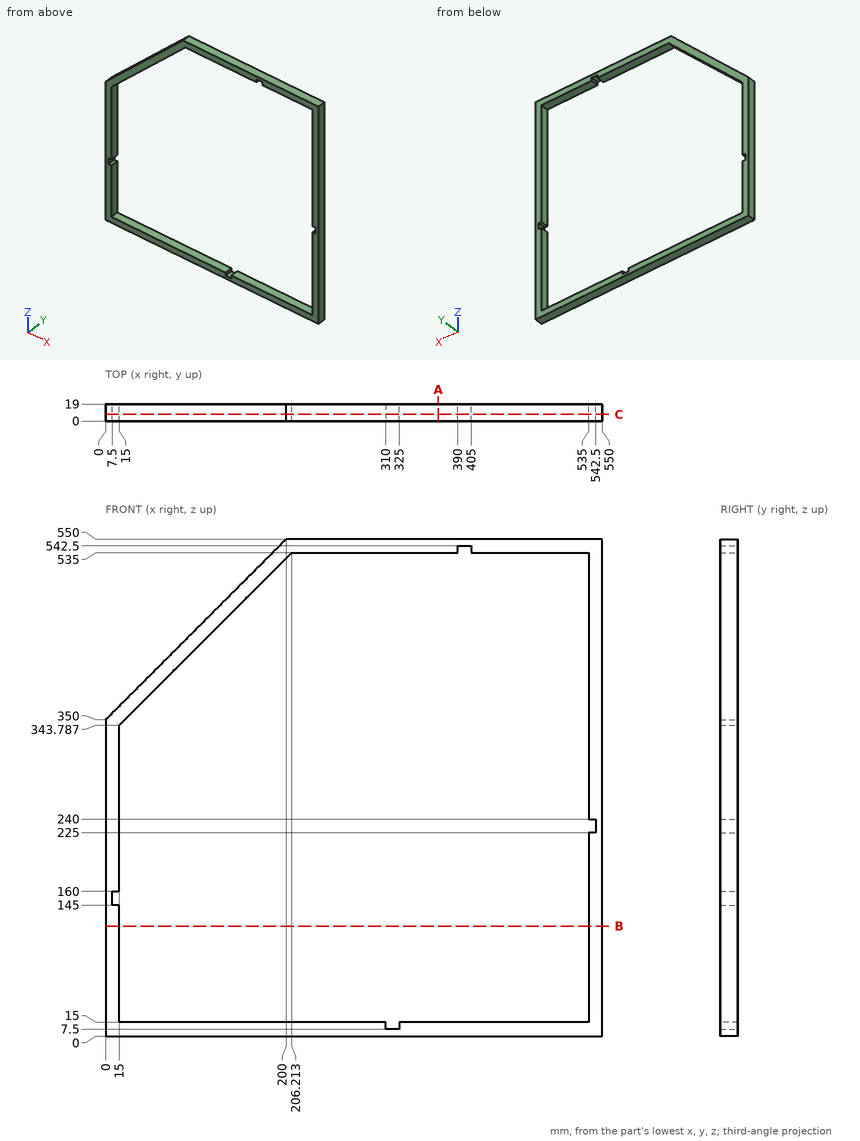
Verification items for this drawing (mm, ordinates from the low corner). Coordinates: 2 decimals unless noted, no trailing zeros. Write each loop counter-clockwise with the first axis right and the second up, starting at its lowest first coordinate (ties: lowest second). Pieces come first, ordered by that corner, then holes. Notation, with made-up numbers: M 40,80 L 46,80 A24 ccw 46,99 Z; hole C 28,19 d2. An arc over 180 degrees is marked long. Answer as a JSON object with one key per item and string values. Group by question number.
(1) Cross-section at B-B, the plane z = 121.5. Record the cut outline in (x, y), and give its area (3 significant figures).
(2) Cross-section at C-C, the plane y = 7.5. Record the cut outline in (x, z), and give its area (3 significant figures).
(3) Gauge pin test, flat ends, axial feed: pin 1 (4 mm diameter, centred on y = 5, z = 539, fed in from -X); pin 2 (9.5 mm diameter, centred on x = 91, y = 9, fed in from +Z); pin 3 (3 mm diameter, centred on x = 143.5, y = 13, fed in from +Z). Record the tip position at first contact, or that the pin passes through.
(4) Material ranges on line 1 (Z direction, x = 256, y = 12.5); line 2 (Z direction, x = 395, y = 8.5), recorded low to high.
(5) Cross-section at A-A, the plane x = 368.5. Record the cut outline in (y, z).
Reply:
{
 "1": {"outline": "M 0,0 L 15,0 L 15,19 L 0,19 Z; M 535,0 L 550,0 L 550,19 L 535,19 Z", "area": "570 mm²"},
 "2": {"outline": "M 0,0 L 550,0 L 550,550 L 200,550 L 0,350 Z; hole M 7.5,145 L 15,145 L 15,15 L 310,15 L 310,7.5 L 325,7.5 L 325,15 L 535,15 L 535,225 L 542.5,225 L 542.5,240 L 535,240 L 535,535 L 405,535 L 405,542.5 L 390,542.5 L 390,535 L 206.21,535 L 15,343.79 L 15,160 L 7.5,160 Z", "area": "29,900 mm²"},
 "3": {"pin 1": "x = 187", "pin 2": "z = 445.75", "pin 3": "z = 495"},
 "4": {"line 1": "0 to 15, 535 to 550", "line 2": "0 to 15, 542.5 to 550"},
 "5": {"outline": "M 0,0 L 19,0 L 19,15 L 0,15 Z; M 0,535 L 19,535 L 19,550 L 0,550 Z"}
}
